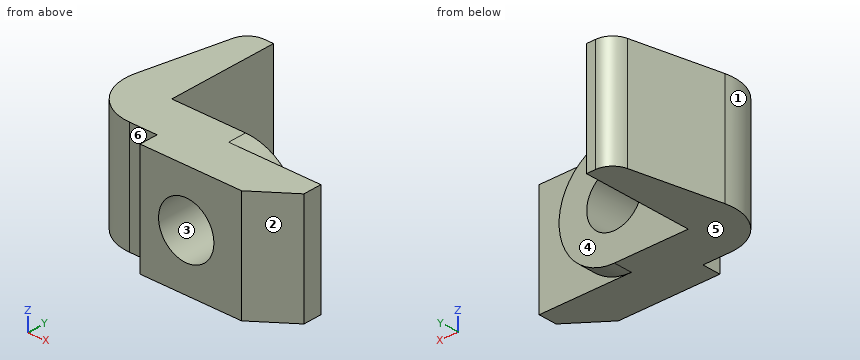
```python
from build123d import *

# Parameters (mm, degrees)
BOSS_EXTRUDE1_DEPTH = 76.2
SKETCH2_R           = 38.1
BOSS_EXTRUDE2_DEPTH = 12.7
SKETCH3_R           = 19.05
CUT_EXTRUDE1_DEPTH  = 45.45
BOSS_EXTRUDE3_DEPTH = 76.2


with BuildPart() as part:
    # Sketch1 → Boss-Extrude1 (new body)
    with BuildSketch(Plane.XY):
        Polygon((0, 0), (69.85, 0), (95.25, 19.05), (95.25, 31.75), (31.75, 31.75), (31.75, 44.45), (-19.05, 44.45), (-19.05, 12.7), (0, 12.7), align=None)
    extrude(amount=BOSS_EXTRUDE1_DEPTH)

    # Sketch2 → Boss-Extrude2 (add, through all)
    with BuildSketch(Plane(origin=(0, 31.75, 0), x_dir=(1, 0, 0), z_dir=(0, 1, 0))):
        with Locations((31.75, -38.1)):
            Circle(SKETCH2_R)
    extrude(amount=BOSS_EXTRUDE2_DEPTH)

    # Sketch3 → Cut-Extrude1 (cut, through all)
    with BuildSketch(Plane(origin=(0, 44.45, 0), x_dir=(1, 0, 0), z_dir=(0, 1, 0))):
        with Locations((31.75, -38.1)):
            Circle(SKETCH3_R)
    extrude(amount=-CUT_EXTRUDE1_DEPTH, mode=Mode.SUBTRACT)

    # Sketch4 → Boss-Extrude3 (add, through all)
    with BuildSketch(Plane.XY.offset(76.2)):
        with BuildLine():
            Line((-19.05, 44.45), (-19.05, 120.65))
            Line((-19.05, 120.65), (-25.4, 120.65))
            ThreePointArc((-25.4, 120.65), (-33.421823369, 117.795829058), (-37.838031752, 110.516196825))
            Line((-37.838031752, 110.516196825), (-50.145079379, 50.865492062))
            ThreePointArc((-50.145079379, 50.865492062), (-43.664572645, 24.395441578), (-19.05, 12.7))
            Line((-19.05, 12.7), (-19.05, 44.45))
        make_face()
    extrude(amount=-BOSS_EXTRUDE3_DEPTH)


solid = part.part
```
Build history of the part. All positions in model axes, mm. Face numbers are marked on the shaded views. A direction names the side the tool comes from. Round coordinates to 2 decimals unless told otherwise and drop trailing zeros. Write each loop counter-clockwise with the first axis right and the second up, starting at its lowest first coordinate (ties: lowest second). Pieces come first, ordered by that corner, then holes. Notation, with made-up numbers: (-28, 25.25) - (-7, 25.25) arc R22 cw to (-7, 41.25) - close; hole circle Ø6 at (63.25, 18). An arc over 180 degrees is marked (long way). Answer as CSV lines item,"result".
Q1. Cut at C-C (y = 22). Write the cut outline in (x, z).
Report:
outline,"(-41.5, 0) - (95.25, 0) - (95.25, 76.2) - (-41.5, 76.2) - close; hole circle Ø38.1 at (31.75, 38.1)"
Q2. Tool access for the marked faces 4, 5 and 6: list every direction of +Z, -Z, +X, -X, +Y, -Y with a clear straight run to the whole face (end or side of a thin tool).
Report:
face 4,"+Z, -Z, +X, +Y"
face 5,"-Z, +X, -X, +Y, -Y"
face 6,"+Z, -Z, -X, -Y"
Q3. Pull direction X, two halves, no side cores. Call the marked faces 1, 2 and 3: +X half, -X half, draft (parallel to the pull), parting line (faces both ways), or undercut.
Report:
face 1,"-X half"
face 2,"+X half"
face 3,"undercut"
Q4. Drop flat-ended pins along their axis: pin 1 (12 mm diameter, centred on x = -8, z = 24, fed in from -Y); pin 2 (1.5 mm diameter, centred on x = 18, z = 20, fed in from +Y); pin 3 (6.5 mm diameter, centred on y = 5, z = 38, fed in from -X). Give the stop position or say it passes through.
Report:
pin 1,"stops at y = 12.7"
pin 2,"stops at y = 44.45"
pin 3,"stops at x = 0"
Q5. Drill centre lines: probe 1 along Z at (x, y) = (31.75, 13); probe 2 along Y at (x, z) = (13, 66.5); probe 3 along X at (y, z) = (25, 38). Where is each one in solid material? Low to high. Write a range as [from, to].
Report:
probe 1,"z = [0, 19.05], [57.15, 76.2]"
probe 2,"y = [0, 44.45]"
probe 3,"x = [-44.15, 12.7], [50.8, 95.25]"
Q6. Cut at B-B (x = 39.5). Write the cut outline in (y, z).
Report:
outline,"(0, 0) - (31.75, 0) - (31.75, 0.8) - (44.45, 0.8) - (44.45, 20.7) - (0, 20.7) - close; (0, 55.5) - (44.45, 55.5) - (44.45, 75.4) - (31.75, 75.4) - (31.75, 76.2) - (0, 76.2) - close"
Q7. Cut at D-D (z = 26). Write the cut outline in (x, y).
Report:
outline,"(-50.15, 50.87) arc R31.75 ccw to (-19.05, 12.7) - (0, 12.7) - (0, 0) - (17.04, 0) - (17.04, 44.45) - (-19.05, 44.45) - (-19.05, 120.65) - (-25.4, 120.65) arc R12.7 ccw to (-37.84, 110.52) - close; (46.46, 0) - (69.85, 0) - (95.25, 19.05) - (95.25, 31.75) - (67.88, 31.75) - (67.88, 44.45) - (46.46, 44.45) - close"
Q8. Cut at A-A (z = 38.1). Write the cut outline in (x, y), and give its area (3 significant figures).
Report:
outline,"(-50.15, 50.87) arc R31.75 ccw to (-19.05, 12.7) - (0, 12.7) - (0, 0) - (12.7, 0) - (12.7, 44.45) - (-19.05, 44.45) - (-19.05, 120.65) - (-25.4, 120.65) arc R12.7 ccw to (-37.84, 110.52) - close; (50.8, 0) - (69.85, 0) - (95.25, 19.05) - (95.25, 31.75) - (69.85, 31.75) - (69.85, 44.45) - (50.8, 44.45) - close"
area,"5,220 mm^2"
